Drawing for the job (mm, zero at the part's lowest x, y, z). Round coordinates to 2 decimals unless told otherwise and drop trailing zeros. Loops run counter-clockwise (first coordinate to the right, second up) from the corner with the lowest first, then second, coordinate; pieces in that order, holes last. Notation, with made-up numbers: M 64.25,15 L 113.25,15 A17 cw 113.25,42 Z; hole C -24,41 d9. An arc over 180 degrees is marked long. Use a Markdown table: item, result. Add a question column.
Q1. Cut at B-B (y = 25). Give the cut face in (x, z), plus the area to 3 significant figures.
Q2. Cut at D-D (x = 168). Give the cut face in (y, z).
Q3. Cut at C-C (y = 16). State how many separate pieces and enclosed holes the cut face has, plus the area to 3 significant figures.
Q4. Mould opens along Y. For the marked faces 1, 2 and 3 say: +Y half, -Y half, draft (parallel to the pull), parting line (faces both ways), or undercut.
Q5. Probe line 1 (Z direction, x = 11, y = 11); line 2 (X direction, y = 28.5, z = 44.5); line 3 (Y direction, x = 155, z = 63.5). List the from-to ranges inside material, lowest first. Write a range as from..to.
Q6. Cut at A-A (z = 34). Give the cut face in (x, y).
Q7. Pin check, flat tips, straight feed: pin 1 (10 mm diameter, centred on y = 26.5, z = 65, fed in from +X); pin 2 (13 mm diameter, centred on x = 169.889, z = 34, fed in from +Y). Stop position of each tip, or through.
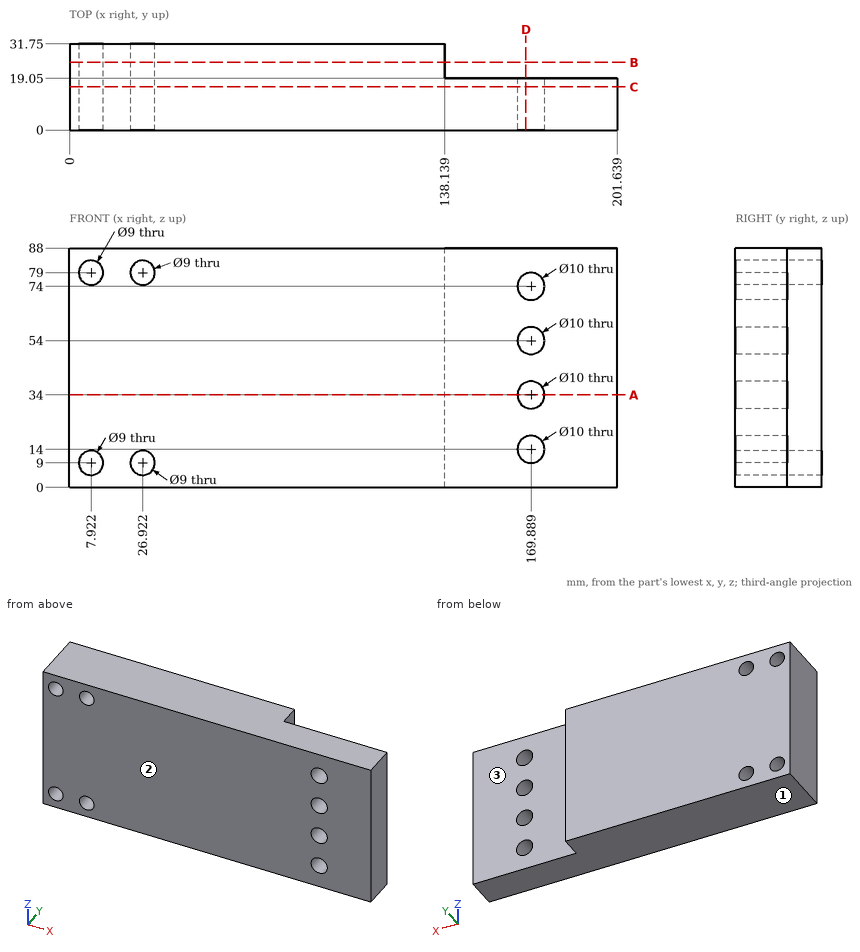
Checked values:
| question | item | result |
|---|---|---|
| 1 | outline | M 0,0 L 138.14,0 L 138.14,88 L 0,88 Z; hole C 7.92,9 d9; hole C 7.92,79 d9; hole C 26.92,9 d9; hole C 26.92,79 d9 |
| 1 | area | 11,900 mm^2 |
| 2 | outline | M 0,0 L 19.05,0 L 19.05,9.37 L 0,9.37 Z; M 0,18.63 L 19.05,18.63 L 19.05,29.37 L 0,29.37 Z; M 0,38.63 L 19.05,38.63 L 19.05,49.37 L 0,49.37 Z; M 0,58.63 L 19.05,58.63 L 19.05,69.37 L 0,69.37 Z; M 0,78.63 L 19.05,78.63 L 19.05,88 L 0,88 Z |
| 3 | separate pieces | 1 |
| 3 | enclosed holes | 8 |
| 3 | area | 17,200 mm^2 |
| 4 | face 1 | draft |
| 4 | face 2 | -Y half |
| 4 | face 3 | +Y half |
| 5 | line 1 | z = 0..5.72, 12.28..75.72, 82.28..88 |
| 5 | line 2 | x = 0..138.14 |
| 5 | line 3 | y = 0..19.05 |
| 6 | outline | M 0,0 L 164.89,0 L 164.89,19.05 L 138.14,19.05 L 138.14,31.75 L 0,31.75 Z; M 174.89,0 L 201.64,0 L 201.64,19.05 L 174.89,19.05 Z |
| 7 | pin 1 | stops at x = 138.14 |
| 7 | pin 2 | stops at y = 19.05 |
